Source: CAD feature listing. Evaluate the final solid. Frame: model axes, mm. Face numbers are marked on the shaded views. Give positions to 0.01 mm unless a question says otherwise; leave off trailing zeros. Order: outer loops, then holes, each group sorted by start corner. A loop starts at its lowest first (then second) coordinate and runs counter-clockwise, first axis right, second up. Notation, with made-up numbers: M -28,5 L 15,5 A29 cw 15,36 Z; hole C 0.5,89 d10. An arc over 180 degrees is marked long. Answer in a Markdown table with one row per item. Add a question column.
(1) Material intervals for line 1 along X through (y, z) = (-4.25, 0); line 2 along Y through (x, z) = (3.5, 27.5) (3 decimals); line 3 along X through (y, z) = (11, -8), sorted ascending.
(2) Pin query (flat end, axial travel): P1, Ø8, axis at y = 5.5, z = -10, coming from the +X side; P2, Ø7.5, axis at x = 7.49, z = 15.78, coming from the +Y side; P3, Ø15, axis at x = 0, z = 0, coming from the +Y side (3 decimals); P4, Ø6, axis at x = 26.5, y = 21, coming from the +Z side. Return the tip coordinate at first contact, or that it passes through.
(3) Section query D-D, the plane y = 13.5. Return loops of the section in (x, z), plus the area to 3 significant figures.
(4) Section query C-C, the plane y = 41.5. Return loops of the section in (x, z).
(5) Mould query, pull axis Z, two halves, no side actions, for the marked faces 1, 2, 3 and 4. Classes: pulls with the +Z half, pulls with the -Z half, needs draft (parallel to the pull), parting line crosses it, or undercut.
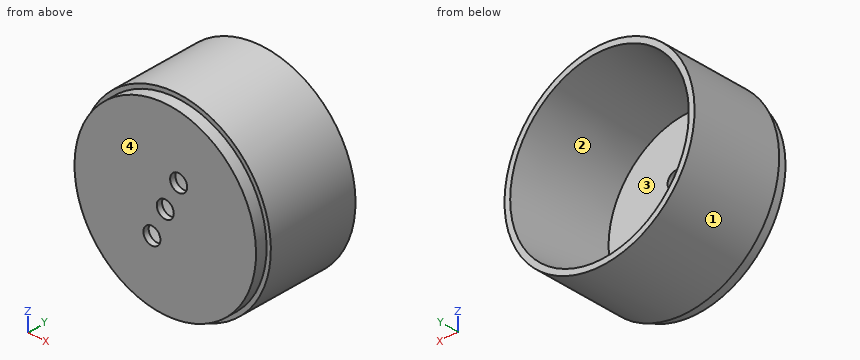
from build123d import *

# Parameters (mm, degrees)
SKETCH1_R           = 53.18125
BOSS_EXTRUDE1_DEPTH = 50.8
SKETCH2_R           = 50.8
SKETCH2_R_2         = 47.625
BOSS_EXTRUDE2_DEPTH = 6.35
SKETCH3_R           = 50.00625
CUT_EXTRUDE1_DEPTH  = 53.975
CUT_EXTRUDE1_DRAFT  = -5
SKETCH4_R           = 4.7625
CUT_EXTRUDE3_DEPTH  = 3.175


with BuildPart() as part:
    # Sketch1 → Boss-Extrude1 (new body)
    with BuildSketch(Plane(origin=(0, 0, 0), x_dir=(1, 0, 0), z_dir=(0, 1, 0))):
        with Locations(Location((0, 0, 0), (0, 0, 270))):
            Circle(SKETCH1_R)
    extrude(amount=BOSS_EXTRUDE1_DEPTH)

    # Sketch2 → Boss-Extrude2 (add)
    with BuildSketch(Plane.XZ):
        with Locations(Location((0, 0, 0), (0, 0, 270))):
            Circle(SKETCH2_R)
        Circle(SKETCH2_R_2, mode=Mode.SUBTRACT)
        Circle(SKETCH2_R_2)
    extrude(amount=BOSS_EXTRUDE2_DEPTH)


with BuildPart() as cut_extrude1_tool:
    # Sketch3 → Cut-Extrude1 (with draft: the straight prism first)
    with BuildSketch(Plane(origin=(0, 50.8, 0), x_dir=(1, 0, 0), z_dir=(0, 1, 0))):
        Circle(SKETCH3_R)
    extrude(amount=-CUT_EXTRUDE1_DEPTH)
    # Cut-Extrude1: the draft: its side faces are tilted about the plane it starts from
    cut_extrude1_sides = [cut_extrude1_tool.faces().sort_by_distance(p)[0] for p in [
        (-50.00625, 23.8125, 0),
    ]]
    draft(cut_extrude1_sides, Plane(origin=(0, 50.8, 0), x_dir=(1, 0, 0), z_dir=(0, 1, 0)), CUT_EXTRUDE1_DRAFT)


with BuildPart() as part_1:
    add(part.part)

    # Cut-Extrude1: cut by cut_extrude1_tool
    add(cut_extrude1_tool.part, mode=Mode.SUBTRACT)

    # Sketch4 → Cut-Extrude3 (cut)
    with BuildSketch(Plane(origin=(0, -3.175, 0), x_dir=(1, 0, 0), z_dir=(0, 1, 0))):
        with Locations(Location((7.487131795, -15.775986934, 0), (0, 0, 270))):
            Circle(SKETCH4_R)
        with Locations(Location((0, 0, 0), (0, 0, 270))):
            Circle(SKETCH4_R)
        with Locations(Location((-7.487131795, 15.775986934, 0), (0, 0, 270))):
            Circle(SKETCH4_R)
    extrude(amount=-CUT_EXTRUDE3_DEPTH, mode=Mode.SUBTRACT)


solid = part_1.part
Values follow:
| question | item | result |
|---|---|---|
| 1 | line 1 | x = -50.8 to -4.76, 4.76 to 50.8 |
| 1 | line 2 | y = -6.35 to -3.175 |
| 1 | line 3 | x = -52.58 to -45.83, 45.83 to 52.58 |
| 2 | P1 | stops at x = 52.84 |
| 2 | P2 | passes through |
| 2 | P3 | stops at y = -3.175 |
| 2 | P4 | stops at z = 47.71 |
| 3 | outline | C 0,0 d106.36; hole C 0,0 d93.49 |
| 3 | area | 2,020 mm² |
| 4 | outline | C 0,0 d106.36; hole C 0,0 d98.39 |
| 5 | face 1 | parting line crosses it |
| 5 | face 2 | undercut |
| 5 | face 3 | undercut |
| 5 | face 4 | needs draft |
